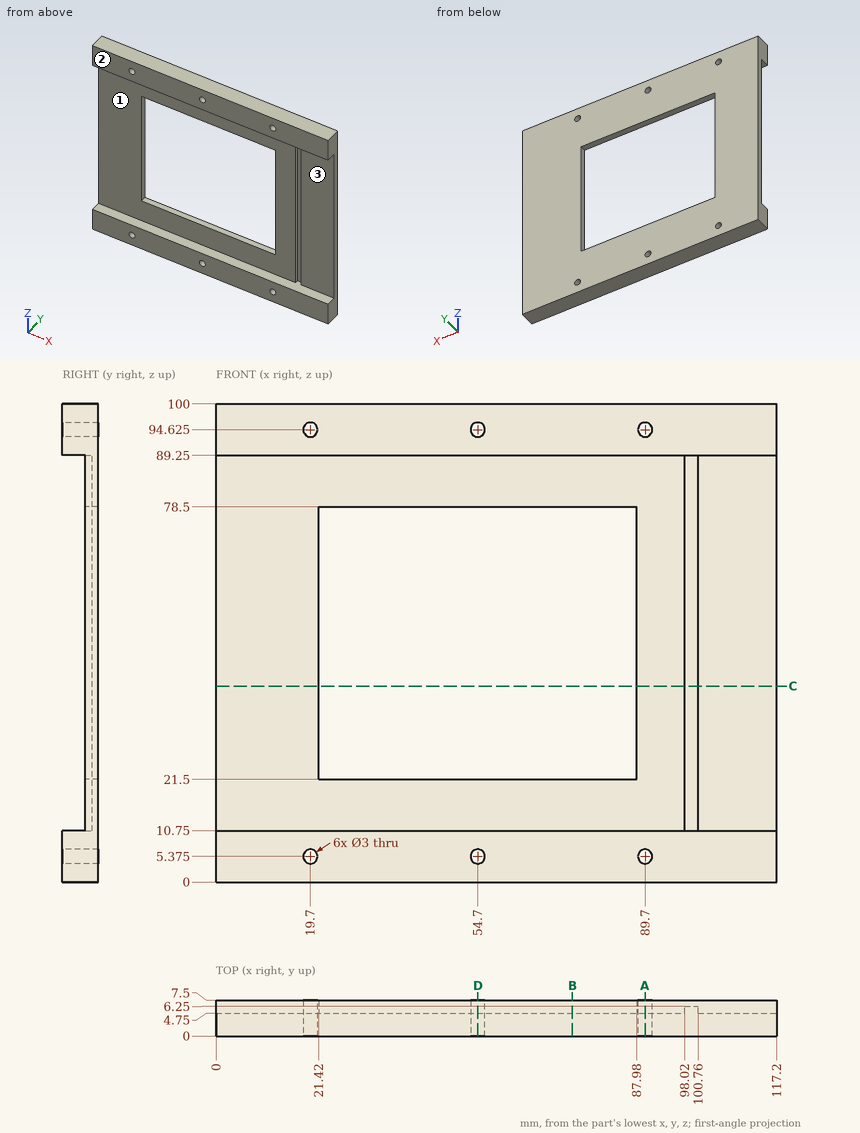
Source: three-view drawing plus pictorial views. Frame: mm from the lowest corner of the part. Coordinates: 2 decimals unless noted, no trailing zeros. Order: outer loops, then holes, each group sorted by start corner. A loop starts at its lowest first (then second) coordinate and runs counter-clockwise, first axis right, second up. Notation, with made-up numbers: M 28.25,45.25 L 83.25,45.25 A28 cw 83.25,75.25 Z; hole C 61.5,-17.5 d11. An arc over 180 degrees is marked long. Answer in a Markdown table with one row per item.
(1) Section query A-A, the plane x = 89.7. Output: boundary loops of the cut face in (y, z) (3 decimals).
Numbers:
| item | result |
|---|---|
| outline | M 0,0 L 7.5,0 L 7.5,3.875 L 0,3.875 Z; M 0,6.875 L 7.5,6.875 L 7.5,93.125 L 0,93.125 L 0,89.25 L 4.75,89.25 L 4.75,10.75 L 0,10.75 Z; M 0,96.125 L 7.5,96.125 L 7.5,100 L 0,100 Z |
(2) Section query D-D, the plane x = 54.7. Output: boundary loops of the cut face in (y, z) (3 decimals).
Numbers:
| item | result |
|---|---|
| outline | M 0,0 L 7.5,0 L 7.5,3.875 L 0,3.875 Z; M 0,6.875 L 7.5,6.875 L 7.5,21.5 L 4.75,21.5 L 4.75,10.75 L 0,10.75 Z; M 0,89.25 L 4.75,89.25 L 4.75,78.5 L 7.5,78.5 L 7.5,93.125 L 0,93.125 Z; M 0,96.125 L 7.5,96.125 L 7.5,100 L 0,100 Z |
(3) Material intervals for line 1 (Z direction, x = 54.7, y = 5.5) (3 decimals); line 2 (Z direction, x = 89.7, y = 2.25) (3 decimals); line 3 (X direction, y = 5.25, z = 68), sorted ascending. Write a range as [from, to].
Numbers:
| item | result |
|---|---|
| line 1 | z = [0, 3.875], [6.875, 21.5], [78.5, 93.125], [96.125, 100] |
| line 2 | z = [0, 3.875], [6.875, 10.75], [89.25, 93.125], [96.125, 100] |
| line 3 | x = [0, 21.42], [87.98, 98.02], [100.76, 117.2] |
(4) Section query B-B, the plane x = 74.5. Output: boundary loops of the cut face in (y, z), plus the area to 3 significant figures.
Numbers:
| item | result |
|---|---|
| outline | M 0,0 L 7.5,0 L 7.5,21.5 L 4.75,21.5 L 4.75,10.75 L 0,10.75 Z; M 0,89.25 L 4.75,89.25 L 4.75,78.5 L 7.5,78.5 L 7.5,100 L 0,100 Z |
| area | 220 mm^2 |
(5) Contact query for flat-ended pins moving along their axis: pin 1 Ø2.5 at (x, z) = (54.7, 5.375) entering from -Y; pin 2 Ø18 at (x, z) = (111, 41) entering from -Y. Output: stop coordinate, or through.
Numbers:
| item | result |
|---|---|
| pin 1 | passes through |
| pin 2 | stops at y = 4.75 |
(6) Section query C-C, the plane z = 41. Output: boundary loops of the cut face in (x, y).
Numbers:
| item | result |
|---|---|
| outline | M 0,4.75 L 21.42,4.75 L 21.42,7.5 L 0,7.5 Z; M 87.98,4.75 L 98.02,4.75 L 98.02,6.25 L 100.76,6.25 L 100.76,4.75 L 117.2,4.75 L 117.2,7.5 L 87.98,7.5 Z |
(7) Draft query along Z for the marked faces 1, 2 and 3. Return one class per face: pulls with the +Z half, pulls with the -Z half, needs draft (parallel to the pull), parting line crosses it, or undercut.
Numbers:
| item | result |
|---|---|
| face 1 | undercut |
| face 2 | needs draft |
| face 3 | undercut |
